Read the model definition and answer for the solid it produces. Units are mm, in the model's axes. Coordinates: 2 decimals unless noted, no trailing zeros. Write each loop counter-clockwise with the first axis right and the second up, starting at its lowest first coordinate (ties: lowest second). Pieces come first, ordered by that corner, then holes. Notation, with made-up numbers: (68.5, -1) -> (104.5, -1) arc R19 cw to (104.5, 14) -> close; hole circle Ø8 at (59.25, 6). An arc over 180 degrees is marked (long way). Use CSV: the item, a comma, the result in double quotes.
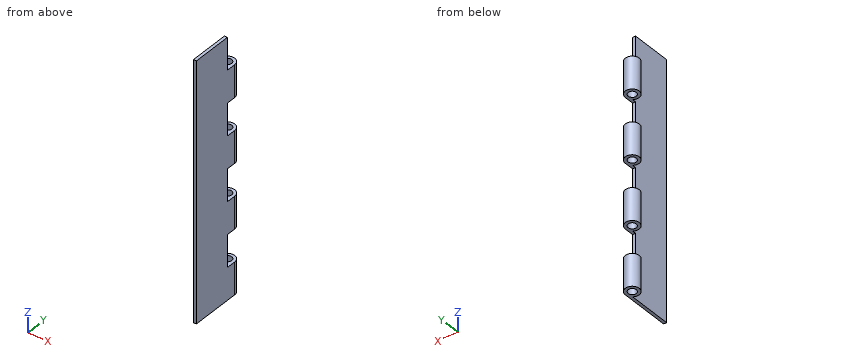
from build123d import *

# Parameters (mm, degrees)
SKETCH1_R           = 3.175
BOSS_EXTRUDE1_DEPTH = 203.2
SKETCH2_W           = 25.4
SKETCH2_H           = 12.7
CUT_EXTRUDE1_DEPTH  = 11.922
LPATTERN1_COUNT     = 4
LPATTERN1_PITCH     = 50.8


with BuildPart() as part:
    # Sketch1 → Boss-Extrude1 (new body)
    with BuildSketch(Plane.XY):
        with BuildLine():
            Line((5.461, 0), (5.461, -38.1))
            Line((5.461, -38.1), (3.175, -38.1))
            Line((3.175, -38.1), (3.175, -4.443185344))
            ThreePointArc((3.175, -4.443185344), (-4.855985791, 2.498384078), (5.461, 0))
        make_face()
        Circle(SKETCH1_R, mode=Mode.SUBTRACT)
    extrude(amount=BOSS_EXTRUDE1_DEPTH)

    # Sketch2 → Cut-Extrude1 (cut, through all)
    with BuildSketch(Plane(origin=(5.461, 0, 0), x_dir=(0, 0, -1), z_dir=(1, 0, 0))):
        with Locations((-190.5, -0.889)):
            Rectangle(SKETCH2_W, SKETCH2_H)
    cut_extrude1 = extrude(amount=-CUT_EXTRUDE1_DEPTH, mode=Mode.SUBTRACT)

    # LPattern1: Cut-Extrude1 ×4
    with Locations(*[(0, 0, -i * LPATTERN1_PITCH) for i in range(1, LPATTERN1_COUNT)]):
        add(cut_extrude1, mode=Mode.SUBTRACT)


solid = part.part
1. A cutting plane is placed at B-B (z = 107.5). Give the vertices of the cut face in (x, y) (3 decimals), and give its area (3 significant figures).
Solutions:
outline,"(3.175, -38.1) -> (5.461, -38.1) -> (5.461, 0) arc R5.461 ccw (long way) to (3.175, -4.443) -> close; hole circle Ø6.35 at (0, 0)"
area,"142 mm^2"
2. A cutting plane is placed at A-A (x = 0). Give the number of separate pieces and of enclosed holes in the cut face, and give its area (3 significant figures).
Solutions:
separate pieces,"8"
enclosed holes,"0"
area,"465 mm^2"
3. A cutting plane is placed at C-C (y = -9). Give the vertices of the cut face in (x, z) (3 decimals), and give its area (3 significant figures).
Solutions:
outline,"(3.175, 0) -> (5.461, 0) -> (5.461, 203.2) -> (3.175, 203.2) -> close"
area,"465 mm^2"
4. Each of these flat-tipped pins is pushed along its axis until it touches: pin 1 Ø2 at (x, y) = (1, -31.5) entering from +Z; pin 2 Ø10 at (y, z) = (-18, 84.5) entering from -X (3 decimals); pin 3 Ø0.7 at (x, z) = (4, 136.5) entering from +Y; pin 4 Ø3.5 at (x, y) = (-2, -3) entering from +Z. Where does it stop, or does it pass through?
Solutions:
pin 1,"passes through"
pin 2,"stops at x = 3.175"
pin 3,"stops at y = -7.24"
pin 4,"stops at z = 177.8"
5. Find the intervals of material crossed by line 1 along Y through (x, z) = (0, 159.25) (3 decimals); line 2 along Y through (x, z) = (-0.5, 120); line 3 along X through (y, z) = (-19, 161) (3 decimals), in increasing order.
Solutions:
line 1,"y = -5.461 to -3.175, 3.175 to 5.461"
line 2,"y = -5.44 to -3.14, 3.14 to 5.44"
line 3,"x = 3.175 to 5.461"
